```python
from build123d import *

# Parameters (mm, degrees)
F0_W     = 174.625
F0_H     = 63.5
F1_DEPTH = 12.7
F2_W     = 6.3549128033
F2_H     = 6.35
F2_W_2   = 6.35
F3_DEPTH = 174.625


with BuildPart() as f1:
    # F0 (on Front) → F1 (new body)
    with BuildSketch(Plane.XZ):
        Rectangle(F0_W, F0_H)
    extrude(amount=F1_DEPTH)

    # F2 (on face) → F3 (cut, through all)
    with BuildSketch(Plane.YZ.offset(87.3125)):
        with Locations((-9.5225435983, 22.225)):
            Rectangle(F2_W, F2_H)
        with Locations((-9.525, -22.225)):
            Rectangle(F2_W_2, F2_H)
    extrude(amount=-F3_DEPTH, mode=Mode.SUBTRACT)


solid = f1.part
```
Source: CAD feature listing. Evaluate the final solid. Frame: model axes, mm. A direction names the side the tool comes from. Give positions to 0.01 mm unless a question says otherwise; leave off trailing zeros. Order: outer loops, then holes, each group sorted by start corner. A loop starts at its lowest first (then second) coordinate and runs counter-clockwise, first axis right, second up.
(1) Pull-direction query (X, two-part tool) for faces 3 (the face through (-1, -12.7, 0)), 4 (the face through (87.312, -6, 0)), 5 (the face through (-87.312, -6, 0)); classes: +X half, -X half, draft (parallel to the pull), parting line (faces both ways), or undercut.
(2) Contact query for a flat-ended pin moving along its axis: P1, Ø1.9, axis at x = 27, z = -23, coming from the -Y side. Output: stop coordinate, or through.
(3) Section query C-C (z = -21). Return the cut outline in (x, y).
(4) Material intervals for line 1 along Z through (x, y) = (-63.5, -8.25); line 2 along Y through (x, z) = (61, -23), sorted ascending.
(5) Access query for faces 1 (the face through (-1, -12.7, 29)), 2 (the face through (1, -10, -19.05)). Directions: +Z, -Z, +X, -X, +Y, -Y. A direction counts if a zero-diameter tool reaches every point of the face in a straight line with its end or side. Return the directions, or none.
(6) Section query A-A (y = -11). Return the cut outline in (x, z).
(7) Section query B-B (x = -18). Return the cut outline in (y, z), plus the area to 3 significant figures.
Outcome:
1. face 3: draft
1. face 4: +X half
1. face 5: -X half
2. P1: stops at y = -6.35
3. outline: (-87.31, -6.35) - (87.31, -6.35) - (87.31, 0) - (-87.31, 0) - close
4. line 1: z = -31.75 to -25.4, -19.05 to 19.05, 25.4 to 31.75
4. line 2: y = -6.35 to 0
5. face 1: +Z, -Z, +X, -X, -Y
5. face 2: +X, -X, -Y
6. outline: (-87.31, -31.75) - (87.31, -31.75) - (87.31, -25.4) - (-87.31, -25.4) - close; (-87.31, -19.05) - (87.31, -19.05) - (87.31, 19.05) - (-87.31, 19.05) - close; (-87.31, 25.4) - (87.31, 25.4) - (87.31, 31.75) - (-87.31, 31.75) - close
7. outline: (-12.7, -31.75) - (0, -31.75) - (0, 31.75) - (-12.7, 31.75) - (-12.7, 25.4) - (-6.35, 25.4) - (-6.35, 19.05) - (-12.7, 19.05) - (-12.7, -19.05) - (-6.35, -19.05) - (-6.35, -25.4) - (-12.7, -25.4) - close
7. area: 726 mm2
